from build123d import *

# Parameters (mm, degrees)
F0_W     = 120
F0_H     = 60
F1_DEPTH = 30
F2_W     = 4.332021
F2_H     = 54.6
F2_W_2   = 4.302548
F3_DEPTH = 1.05


with BuildPart() as f1:
    # F0 (on Front) → F1 (new body, symmetric)
    with BuildSketch(Plane.XZ):
        Rectangle(F0_W, F0_H)
    extrude(amount=F1_DEPTH, both=True)

    # F2 (on Front) → F3 (join, symmetric)
    with BuildSketch(Plane.XZ):
        Polygon((59.720043, 27.3), (60, 27.3), (60, 30.02), (-60, 30.02), (-60, 27.3), (-55.697452, 27.3), (55.388022, 27.3), align=None)
        with Locations((57.554032, 0)):
            Rectangle(F2_W, F2_H)
        Polygon((60, -27.3), (59.720043, -27.3), (55.388022, -27.3), (-55.697452, -27.3), (-60, -27.3), (-60, -30.02), (60, -30.02), align=None)
        with Locations((-57.848726, 0)):
            Rectangle(F2_W_2, F2_H)
    extrude(amount=F3_DEPTH, both=True)


solid = f1.part
Design review of the part built by this model. Coordinates are the model's own, in mm. Give positions to 0.01 mm unless a question says otherwise; leave off trailing zeros. One line per question, with ' | ' between items. Start each with the question number.
(1) Insertion check: P1, Ø8.5, axis at x = 22.5, y = 13, coming from the -Z side; P2, Ø10, axis at x = 22.5, y = -13.5, coming from the +Z side. Each pin has a flat end and moves straight along its axis. Give the tip position at first contact, or say it passes through.
(2) Draft analysis for pull direction Y (two halves, no side actions). For faces 1 (the face through (-1, 15, 30)), 2 (the face through (-1, -30, 0)), 3 (the face through (-1, 30, 0)), state which applies: +Y half, -Y half, draft (parallel to the pull), parting line (faces both ways), or undercut.
(3) For line 1 (Z direction, x = -21, y = -17), list the stretches that pass through material, from the lowest coordinate up.
The answers:
1) P1: stops at z = -30 | P2: stops at z = 30
2) face 1: draft | face 2: -Y half | face 3: +Y half
3) line 1: z = -30 to 30
